Design review of the part built by this model. Coordinates are the model's own, in mm. Round coordinates to 2 decimals unless told otherwise and drop trailing zeros. Order: outer loops, then holes, each group sorted by start corner. A loop starts at its lowest first (then second) coordinate and runs counter-clockwise, first axis right, second up. Notation, with made-up numbers: (40, 39.25) - (50, 39.25) arc R23 cw to (50, 49.25) - close; hole circle Ø7 at (30.5, 89). An arc over 180 degrees is marked (long way). Use CSV: the item, a comma, the result in double quotes.
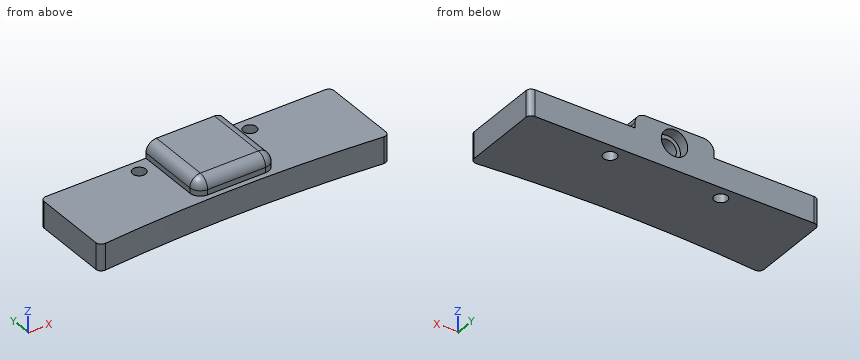
from build123d import *

# Parameters (mm, degrees)
BOSS_EXTRUDE1_DEPTH                     = 5
SKETCH4_W                               = 15
SKETCH4_H                               = 14
BOSS_EXTRUDE2_DEPTH                     = 3
CBORE_FOR_M6_HEX_HEAD_BOLT1_D           = 3.5
CBORE_FOR_M6_HEX_HEAD_BOLT1_DEPTH       = 10
CBORE_FOR_M6_HEX_HEAD_BOLT1_CBORE_D     = 5
CBORE_FOR_M6_HEX_HEAD_BOLT1_CBORE_DEPTH = 2
CBORE_FOR_M6_HEX_HEAD_BOLT1_TIP         = 1.75
FILLET1_R                               = 1
FILLET2_R                               = 2
M3X0_5_TAPPED_HOLE1_D                   = 2.5
M3X0_5_TAPPED_HOLE1_DEPTH               = 5
M3X0_5_TAPPED_HOLE1_TIP                 = 0.751075774


with BuildPart() as part:
    # Sketch1 → Boss-Extrude1 (new body)
    with BuildSketch(Plane(origin=(0, 0, 0), x_dir=(-1, 0, 0), z_dir=(0, 0, -1))):
        with BuildLine():
            Line((27.500000074, -16.263075607), (27.500000074, 0))
            Line((27.500000074, 0), (-27.5, 0))
            Line((-27.5, 0), (-27.5, -16.2630756))
            ThreePointArc((-27.5, -16.2630756), (3.7e-08, -15), (27.500000074, -16.263075607))
        make_face()
    extrude(amount=-BOSS_EXTRUDE1_DEPTH)

    # Sketch4 → Boss-Extrude2 (add)
    with BuildSketch(Plane.XY.offset(5)):
        with Locations((0, -7)):
            Rectangle(SKETCH4_W, SKETCH4_H)
    extrude(amount=BOSS_EXTRUDE2_DEPTH)

    # CBORE for M6 Hex Head Bolt1
    with Locations(Plane(origin=(0, 0, 0), x_dir=(1, 0, 0), z_dir=(0, 1, 0))):
        with Locations((0, -5)):
            CounterBoreHole(CBORE_FOR_M6_HEX_HEAD_BOLT1_D / 2, CBORE_FOR_M6_HEX_HEAD_BOLT1_CBORE_D / 2, CBORE_FOR_M6_HEX_HEAD_BOLT1_CBORE_DEPTH, depth=CBORE_FOR_M6_HEX_HEAD_BOLT1_DEPTH)
            with Locations((0, 0, -(CBORE_FOR_M6_HEX_HEAD_BOLT1_DEPTH + CBORE_FOR_M6_HEX_HEAD_BOLT1_TIP / 2))):  # 90° drill point
                Cone(0, CBORE_FOR_M6_HEX_HEAD_BOLT1_D / 2, CBORE_FOR_M6_HEX_HEAD_BOLT1_TIP, mode=Mode.SUBTRACT)

    # Fillet1
    fillet1_edges = [part.edges().sort_by_distance(p)[0] for p in [
        (27.5, 0, 2.5),
        (-27.500000074, 0, 2.5),
        (27.5, -16.2630756, 2.5),
        (-27.500000074, -16.263075607, 2.5),
    ]]
    fillet(fillet1_edges, radius=FILLET1_R)

    # Fillet2
    fillet2_edges = [part.edges().sort_by_distance(p)[0] for p in [
        (7.5, -14, 6.5),
        (7.5, -7, 8),
        (-7.5, -14, 6.5),
        (0, -14, 8),
        (-7.5, -7, 8),
    ]]
    fillet(fillet2_edges, radius=FILLET2_R)

    # M3x0.5 Tapped Hole1
    with Locations(Plane(origin=(-10.5, -2.5, 5), x_dir=(1, 0, 0), z_dir=(0, 0, 1))):
        with Locations((0, 0), (21, 0)):
            Hole(M3X0_5_TAPPED_HOLE1_D / 2, depth=M3X0_5_TAPPED_HOLE1_DEPTH)
            with Locations((0, 0, -(M3X0_5_TAPPED_HOLE1_DEPTH + M3X0_5_TAPPED_HOLE1_TIP / 2))):  # 118° drill point
                Cone(0, M3X0_5_TAPPED_HOLE1_D / 2, M3X0_5_TAPPED_HOLE1_TIP, mode=Mode.SUBTRACT)


solid = part.part
1) We need section A-A (z = 0.5). Give the boundary of the cut face in (x, y), then the cut area to 3 significant figures.
Data:
outline,"(-27.5, -15.17) arc R1 ccw to (-26.41, -16.16) arc R300 cw to (26.41, -16.16) arc R1 ccw to (27.5, -15.17) - (27.5, -1) arc R1 ccw to (26.5, 0) - (-26.5, 0) arc R1 ccw to (-27.5, -1) - close; hole circle Ø2.5 at (-10.5, -2.5); hole circle Ø2.5 at (10.5, -2.5)"
area,"837 mm2"
2) To check wall thickness, follow L1, parallel to Z at x = -24.5, y = -8.25; L2, parallel to X at y = -1.75, z = 5.5; L3, parallel to Y at x = 10.5, z = 1.9. State the ranges of each line that lie inside material, in increasing order. Write a range as from..to.
Data:
L1,"z = 0..5"
L2,"x = -7.5..-2.45, 2.45..7.5"
L3,"y = -15.18..-3.75, -1.25..0"
3) We need section C-C (x = -10.5). Give the boundary of the cut face in (y, z), then the cut area to 3 significant figures.
Data:
outline,"(-15.18, 0) - (-3.75, 0) - (-3.75, 5) - (-15.18, 5) - close; (-1.25, 0) - (0, 0) - (0, 5) - (-1.25, 5) - close"
area,"63.4 mm2"
4) We need section D-D (y = -12.75). Give the boundary of the cut face in (x, z), then the cut area to 3 significant figures.
Data:
outline,"(-27.5, 0) - (27.5, 0) - (27.5, 5) - (7.35, 5) - (7.35, 6) arc R1.85 ccw to (5.5, 7.85) - (-5.5, 7.85) arc R1.85 ccw to (-7.35, 6) - (-7.35, 5) - (-27.5, 5) - close"
area,"316 mm2"
5) Insertion check: pin 1 Ø3 at (x, z) = (0, 5) entering from -Y; pin 2 Ø1.5 at (x, z) = (0.5, 6) entering from +Y; pin 3 Ø0.5 at (y, z) = (-8.5, 5.5) entering from -X; pin 4 Ø2 at (x, y) = (-10.5, -2.5) entering from +Z. Each pin has a flat end and moves straight along its axis. Give the tip position at first contact, or say it passes through.
Data:
pin 1,"stops at y = -15"
pin 2,"stops at y = -2"
pin 3,"stops at x = -7.5"
pin 4,"passes through"
6) We need section B-B (y = -8.5). Give the boundary of the cut face in (x, z).
Data:
outline,"(-27.5, 0) - (27.5, 0) - (27.5, 5) - (7.5, 5) - (7.5, 6) arc R2 ccw to (5.5, 8) - (-5.5, 8) arc R2 ccw to (-7.5, 6) - (-7.5, 5) - (-27.5, 5) - close; hole circle Ø3.5 at (0, 5)"
